```python
from build123d import *

# Parameters (mm, degrees)
SKETCH1_R                      = 4
BOSS_EXTRUDE1_DEPTH            = 3
SKETCH2_R                      = 5.5
BOSS_EXTRUDE2_DEPTH            = 3
CBORE_FOR_M3_SHCS1_D           = 3.4
CBORE_FOR_M3_SHCS1_CBORE_D     = 6.5
CBORE_FOR_M3_SHCS1_CBORE_DEPTH = 3
CHAMFER1_SIZE                  = 1


with BuildPart() as part:
    # Sketch1 → Boss-Extrude1 (new body)
    with BuildSketch(Plane.XY):
        Circle(SKETCH1_R)
    extrude(amount=BOSS_EXTRUDE1_DEPTH)

    # Sketch2 → Boss-Extrude2 (add)
    with BuildSketch(Plane.XY.offset(3)):
        Circle(SKETCH2_R)
    extrude(amount=BOSS_EXTRUDE2_DEPTH)

    # CBORE for M3 SHCS1 (through all)
    with Locations(Plane.XY.offset(6)):
        with Locations((0, 0)):
            CounterBoreHole(CBORE_FOR_M3_SHCS1_D / 2, CBORE_FOR_M3_SHCS1_CBORE_D / 2, CBORE_FOR_M3_SHCS1_CBORE_DEPTH)

    # Chamfer1
    chamfer1_edges = [part.edges().sort_by_distance(p)[0] for p in [
        (-5.5, 0, 6),
    ]]
    chamfer(chamfer1_edges, length=CHAMFER1_SIZE)


solid = part.part
```
Part model, mm, in its own coordinate system. A direction names the side the tool comes from. Round coordinates to 2 decimals unless told otherwise and drop trailing zeros. Order: outer loops, then holes, each group sorted by start corner. A loop starts at its lowest first (then second) coordinate and runs counter-clockwise, first axis right, second up. Notation, with made-up numbers: M 70,-34.75 L 126,-34.75 A15 ccw 126,-18.75 Z; hole C 8,63 d3. An arc over 180 degrees is marked long. Put each result on its own line as item: value. Start each with the question number.
1. Two-plate mould, pull along X, no slides. Class faces 1 (the face through (3, -2, 6)), 2 (the face through (-1.19, -5.37, 3.99)), 3 (the face through (1.4, -1.4, 3)), 4 (the face through (-2.579, -1.978, 4.521)): +X half, -X half, draft (parallel to the pull), parting line (faces both ways), or undercut.
2. Slice it at D-D on z = 4.6. List the corners of the cut face in (x, y), then the cut area to 4 significant figures.
3. Slice it at C-C on z = 1.75. List the corners of the cut face in (x, y).
4. Slice it at A-A on y = 0. List the corners of the cut face in (x, z).
5. Drill centre lines: probe 1 along Y at (x, z) = (0, 4.05); probe 2 along Y at (x, z) = (0, 1.95); probe 3 along X at (y, z) = (-3, 5.7). Where is each one in solid material? Low to high. Write a range as [from, to].
6. Drop flat-ended pins along their axis: pin 1 (1.5 mm diameter, centred on y = 2.5, z = 1, fed in from +X); pin 2 (1 mm diameter, centred on x = -1.5, y = -0.5, fed in from +Z). Give the stop position or say it passes through.
7. Tool access for faces 5 (the face through (-0.867, -3.905, 1.479)), 6 (the face through (2, 0, 0)): list every direction of +Z, -Z, +X, -X, +Y, -Y with a clear straight run to the whole face (end or side of a thin tool).
Findings:
1. face 1: draft
1. face 2: parting line
1. face 3: undercut
1. face 4: undercut
2. outline: C 0,0 d11; hole C 0,0 d6.5
2. area: 61.85 mm2
3. outline: C 0,0 d8; hole C 0,0 d3.4
4. outline: M -5.5,3 L -4,3 L -4,0 L -1.7,0 L -1.7,3 L -3.25,3 L -3.25,6 L -4.5,6 L -5.5,5 Z; M 1.7,0 L 4,0 L 4,3 L 5.5,3 L 5.5,5 L 4.5,6 L 3.25,6 L 3.25,3 L 1.7,3 Z
5. probe 1: [-5.5, -3.25], [3.25, 5.5]
5. probe 2: [-4, -1.7], [1.7, 4]
5. probe 3: [-3.75, -1.25], [1.25, 3.75]
6. pin 1: x = 3.6
6. pin 2: z = 3
7. face 5: -Z
7. face 6: -Z, +X, -X, +Y, -Y
